from build123d import *

# Parameters (mm, degrees)
SKETCH1_W           = 101.6
SKETCH1_H           = 50.8
BOSS_EXTRUDE1_DEPTH = 3.175
SKETCH3_W           = 101.6
SKETCH3_H           = 3.175
BOSS_EXTRUDE2_DEPTH = 22.225
SKETCH4_R           = 1.778
CUT_EXTRUDE1_DEPTH  = 117.397422652
SKETCH4_3_R         = 1.778
CUT_EXTRUDE2_DEPTH  = 22.225
SKETCH7_W           = 101.6
SKETCH7_H           = 3.175
CUT_EXTRUDE3_DEPTH  = 25.4


with BuildPart() as part:
    # Sketch1 → Boss-Extrude1 (new body)
    with BuildSketch(Plane(origin=(0, 0, 0), x_dir=(1, 0, 0), z_dir=(0, 1, 0))):
        with Locations((50.8, 25.4)):
            Rectangle(SKETCH1_W, SKETCH1_H)
    extrude(amount=BOSS_EXTRUDE1_DEPTH)

    # Sketch3 → Boss-Extrude2 (add)
    with BuildSketch(Plane(origin=(0, 3.175, 0), x_dir=(1, 0, 0), z_dir=(0, 1, 0))):
        with Locations((50.8, 49.2125)):
            Rectangle(SKETCH3_W, SKETCH3_H)
    extrude(amount=BOSS_EXTRUDE2_DEPTH)

    # Sketch4 → Cut-Extrude1 (cut, through all)
    with BuildSketch(Plane(origin=(0, 0, 0), x_dir=(-1, 0, 0), z_dir=(0, -1, 0))):
        with Locations(Location((-25.4, 31.75, 0), (0, 0, 90))):
            Circle(SKETCH4_R)
    extrude(amount=-CUT_EXTRUDE1_DEPTH, mode=Mode.SUBTRACT)

    # Sketch4_3 → Cut-Extrude2 (cut)
    with BuildSketch(Plane(origin=(0, 0, 0), x_dir=(-1, 0, 0), z_dir=(0, -1, 0))):
        with Locations(Location((-25.4, 31.75, 0), (0, 0, 90))):
            Circle(SKETCH4_3_R)
        with Locations(Location((-76.2, 31.75, 0), (0, 0, 90))):
            Circle(SKETCH4_3_R)
    extrude(amount=-CUT_EXTRUDE2_DEPTH, mode=Mode.SUBTRACT)

    # Sketch7 → Cut-Extrude3 (cut)
    with BuildSketch(Plane.XY):
        with Locations((50.8, 1.5875)):
            Rectangle(SKETCH7_W, SKETCH7_H)
    extrude(amount=-CUT_EXTRUDE3_DEPTH, mode=Mode.SUBTRACT)


solid = part.part
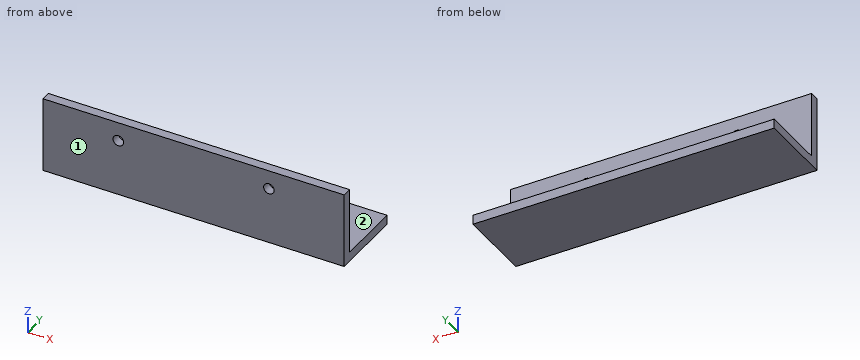
Design review of the part built by this model. Coordinates are the model's own, in mm. Face numbers are marked on the shaded views. A direction names the side the tool comes from. Round coordinates to 2 decimals unless told otherwise and drop trailing zeros. Order: outer loops, then holes, each group sorted by start corner. A loop starts at its lowest first (then second) coordinate and runs counter-clockwise, first axis right, second up. Notation, with made-up numbers: M 14.25,52.25 L 38.25,52.25 A9 cw 38.25,59.25 Z; hole C 72,-20 d4. An arc over 180 degrees is marked long. Answer as CSV lines item,"result". Start each with the question number.
1) Add section D-D (z = -44.75). Give the boundary of the cut face in (x, y) (3 decimals), then the cut area to 3 significant figures.
2) Add section C-C (x = 41). Give the boundary of the cut face in (y, z) (3 decimals), then the cut area to 3 significant figures.
3) Tool access review of the marked faces 1 and 2: name each direction out of +Z, -Z, +X, -X, +Y, -Y from which nothing blocks a thin tool from reaching the whole face with its end or side.
4) Add section B-B (x = 25.4). Give the boundary of the cut face in (y, z) (3 decimals), then the cut area to 3 significant figures.
5) Add section A-A (z = -31.75). Give the boundary of the cut face in (x, y) (3 decimals).
6) For pin 1 Ø4 at (x, z) = (76.2, -31.75) entering from +Y (3 decimals); pin 2 Ø2 at (x, y) = (89.5, 6) entering from +Z (3 decimals), all flat-tipped, find the tip position at first contact; note any pin that passes through.
7) Wall thickness on line 1 along X through (y, z) = (2.2, -31.75); line 2 along Z through (x, y) = (76.2, 0.8); line 3 along Y through (x, z) = (90, -30.25) (3 decimals): over which ranges is each line inside the solid? List them lowest first. Write a range as [from, to].
Resolved:
1,outline,"M 0,0 L 101.6,0 L 101.6,3.175 L 0,3.175 Z"
1,area,"323 mm^2"
2,outline,"M 0,-50.8 L 25.4,-50.8 L 25.4,-47.625 L 3.175,-47.625 L 3.175,-25.4 L 0,-25.4 Z"
2,area,"151 mm^2"
3,face 1,"+Z, -Z, +X, -X, -Y"
3,face 2,"+Z, +X, -X, +Y"
4,outline,"M 0,-50.8 L 25.4,-50.8 L 25.4,-47.625 L 3.175,-47.625 L 3.175,-33.528 L 0,-33.528 Z; M 0,-29.972 L 3.175,-29.972 L 3.175,-25.4 L 0,-25.4 Z"
4,area,"140 mm^2"
5,outline,"M 0,0 L 23.622,0 L 23.622,3.175 L 0,3.175 Z; M 27.178,0 L 74.422,0 L 74.422,3.175 L 27.178,3.175 Z; M 77.978,0 L 101.6,0 L 101.6,3.175 L 77.978,3.175 Z"
6,pin 1,"y = 3.175"
6,pin 2,"z = -47.625"
7,line 1,"[0, 23.62], [27.18, 74.42], [77.98, 101.6]"
7,line 2,"[-50.8, -33.53], [-29.97, -25.4]"
7,line 3,"[0, 3.175]"
